Part model, mm, in its own coordinate system. Face numbers are marked on the shaded views. Give positions to 0.01 mm unless a question says otherwise; leave off trailing zeros. Order: outer loops, then holes, each group sorted by start corner. A loop starts at its lowest first (then second) coordinate and runs counter-clockwise, first axis right, second up.
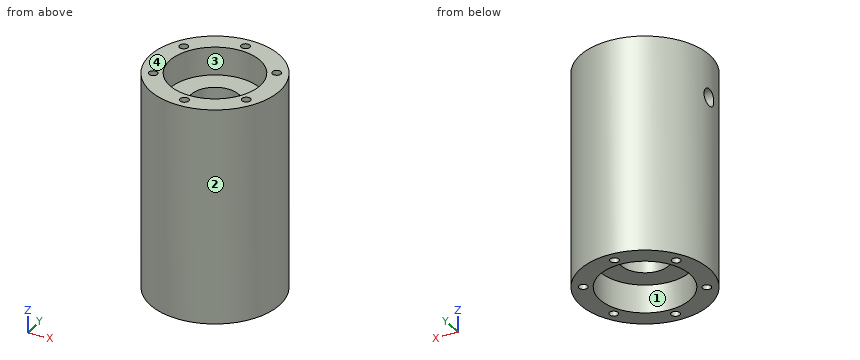
from build123d import *

# Parameters (mm, degrees)
F0_R      = 30
F0_R_2    = 11
F1_DEPTH  = 100
F2_R      = 21
F2_R_2    = 11
F3_DEPTH  = 13
F4_R      = 21
F4_R_2    = 11
F5_DEPTH  = 13
F7_D      = 8
F7_DEPTH  = 30.001
F9_D      = 4
F9_DEPTH  = 30
F9_TIP    = 1.2017212381
F11_D     = 4
F11_DEPTH = 30
F11_TIP   = 1.2017212381


with BuildPart() as f1:
    # F0 (on Top) → F1 (new body)
    with BuildSketch(Plane.XY):
        Circle(F0_R)
        Circle(F0_R_2, mode=Mode.SUBTRACT)
    extrude(amount=F1_DEPTH)

    # F2 (on face) → F3 (cut)
    with BuildSketch(Plane.XY.offset(100)):
        Circle(F2_R)
        Circle(F2_R_2, mode=Mode.SUBTRACT)
    extrude(amount=-F3_DEPTH, mode=Mode.SUBTRACT)

    # F4 (on face) → F5 (cut)
    with BuildSketch(Plane(origin=(0, 0, 0), x_dir=(1, 0, 0), z_dir=(0, 0, -1))):
        Circle(F4_R)
        Circle(F4_R_2, mode=Mode.SUBTRACT)
    extrude(amount=-F5_DEPTH, mode=Mode.SUBTRACT)

    # F7 (through all, one way)
    with BuildSketch(Plane.YZ):
        with Locations((0, 80)):
            Circle(F7_D / 2)
    extrude(amount=-F7_DEPTH, mode=Mode.SUBTRACT)

    # F9
    with Locations(Plane.XY.offset(100)):
        with Locations((0, 25), (21.6506350946, 12.5), (21.6506350946, -12.5), (0, -25), (-21.6506350946, -12.5), (-21.6506350946, 12.5)):
            Hole(F9_D / 2, depth=F9_DEPTH)
            with Locations((0, 0, -(F9_DEPTH + F9_TIP / 2))):  # 118° drill point
                Cone(0, F9_D / 2, F9_TIP, mode=Mode.SUBTRACT)

    # F11
    with Locations(Plane(origin=(0, 0, 0), x_dir=(1, 0, 0), z_dir=(0, 0, -1))):
        with Locations((0, 25), (21.6506350946, 12.5), (21.6506350946, -12.5), (0, -25), (-21.6506350946, -12.5), (-21.6506350946, 12.5)):
            Hole(F11_D / 2, depth=F11_DEPTH)
            with Locations((0, 0, -(F11_DEPTH + F11_TIP / 2))):  # 118° drill point
                Cone(0, F11_D / 2, F11_TIP, mode=Mode.SUBTRACT)


solid = f1.part
Item 1: Band-saw the part on A-A on z = 16. List the corners of the cut face in (x, y).
Item 2: Band-saw the part on D-D on x = 7. List the corners of the cut face in (y, z).
Item 3: Drill centre lines: probe 1 along Y at (x, z) = (0, 20); probe 2 along Y at (x, z) = (21, 26); probe 3 along Y at (x, z) = (0, 3). Where is each one in solid material? Low to high.
Item 4: Drop flat-ended pins along their axis: P1, Ø3, axis at x = 21.65, y = -12.5, coming from the +Z side; P2, Ø2.5, axis at x = 21.65, y = -12.5, coming from the -Z side; P3, Ø3, axis at x = -21.65, y = 12.5, coming from the -Z side. Give the stop position or say it passes through.
Item 5: Pull direction X, two halves, no side cores. Call the marked faces 1, 2, 3 and 4: released by +X, released by -X, zero draft, split by the parting line, or undercut.
Item 6: Band-saw the part on C-C on y = 9. List the corners of the cut face in (x, z).
Item 7: Band-saw the part on B-B on y = 0. List the corners of the cut face in (x, z), plus the area to 3 significant figures.
Working result:
1. outline: circle Ø60 at (0, 0); hole circle Ø4 at (-21.65, -12.5); hole circle Ø4 at (-21.65, 12.5); hole circle Ø22 at (0, 0); hole circle Ø4 at (0, -25); hole circle Ø4 at (0, 25); hole circle Ø4 at (21.65, -12.5); hole circle Ø4 at (21.65, 12.5)
2. outline: (-29.17, 0) - (-19.8, 0) - (-19.8, 13) - (-8.49, 13) - (-8.49, 87) - (-19.8, 87) - (-19.8, 100) - (-29.17, 100) - close; (8.49, 13) - (19.8, 13) - (19.8, 0) - (29.17, 0) - (29.17, 100) - (19.8, 100) - (19.8, 87) - (8.49, 87) - close
3. probe 1: y = -30 to -27, -23 to -11, 11 to 23, 27 to 30
3. probe 2: y = -21.42 to -14.39, -10.61 to 10.61, 14.39 to 21.42
3. probe 3: y = -30 to -27, -23 to -21, 21 to 23, 27 to 30
4. P1: stops at z = 69.7
4. P2: stops at z = 30.45
4. P3: stops at z = 30.3
5. face 1: undercut
5. face 2: split by the parting line
5. face 3: undercut
5. face 4: zero draft
6. outline: (-28.62, 0) - (-18.97, 0) - (-18.97, 13) - (-6.32, 13) - (-6.32, 87) - (-18.97, 87) - (-18.97, 100) - (-28.62, 100) - close; (6.32, 13) - (18.97, 13) - (18.97, 0) - (28.62, 0) - (28.62, 100) - (18.97, 100) - (18.97, 87) - (6.32, 87) - close
7. outline: (-30, 0) - (-21, 0) - (-21, 13) - (-11, 13) - (-11, 76) - (-30, 76) - close; (-30, 84) - (-11, 84) - (-11, 87) - (-21, 87) - (-21, 100) - (-30, 100) - close; (11, 13) - (21, 13) - (21, 0) - (30, 0) - (30, 100) - (21, 100) - (21, 87) - (11, 87) - close
7. area: 3,130 mm2
